Check sheet for the drawn part. Datum: minimum x, y, z corner. Units: mm. A direction names the side the tool comes from. Coordinates: 2 decimals unless noted, no trailing zeros. Write each loop counter-clockwise with the first axis right and the second up, starting at its lowest first coordinate (ties: lowest second). Pieces come first, ordered by that corner, then holes. Notation, with made-up numbers: (47.5, -24.5) -> (77.5, -24.5) arc R18 ccw to (77.5, -10.5) -> close; hole circle Ø4 at (21.5, 80.5). An arc over 180 degrees is marked (long way). Write item = value, one per line. Start each with the question number.
(1) Set-up check for the marked faces 5, 6 and 7: record each of +Z, -Z, +X, -X, +Y, -Y from which the full face is reachable in a straight line by a thin tool's end or side.
(2) Section check A-A (y = 0.75). Record the cut outline in (x, z), plus the area to 3 significant figures.
(3) Mould release check, pull along X, two halves, no side actions. Record for the marked faces 1, 2, 3 and 4: released by +X, released by -X, zero draft, split by the parting line, or undercut.
(4) Gauge pin test, flat ends, axial feed: pin 1 Ø1.5 at (x, z) = (12, 3) entering from -Y; pin 2 Ø0.9 at (y, z) = (1, 4.5) entering from +X; pin 3 Ø1.5 at (y, z) = (1.5, 3) entering from -X. Record the tip position at first contact, or that the pin passes through.
(5) Section check B-B (z = 4.5). Record the cut outline in (x, y), plus the area to 3 significant figures.
(6) Material ranges on probe 1 along X at (y, z) = (1.05, 7.25); probe 2 along Y at (x, z) = (11.5, 1), recorded low to high. Write a range as [from, to].
(7) Section check C-C (x = 13.5). Record the cut outline in (y, z).
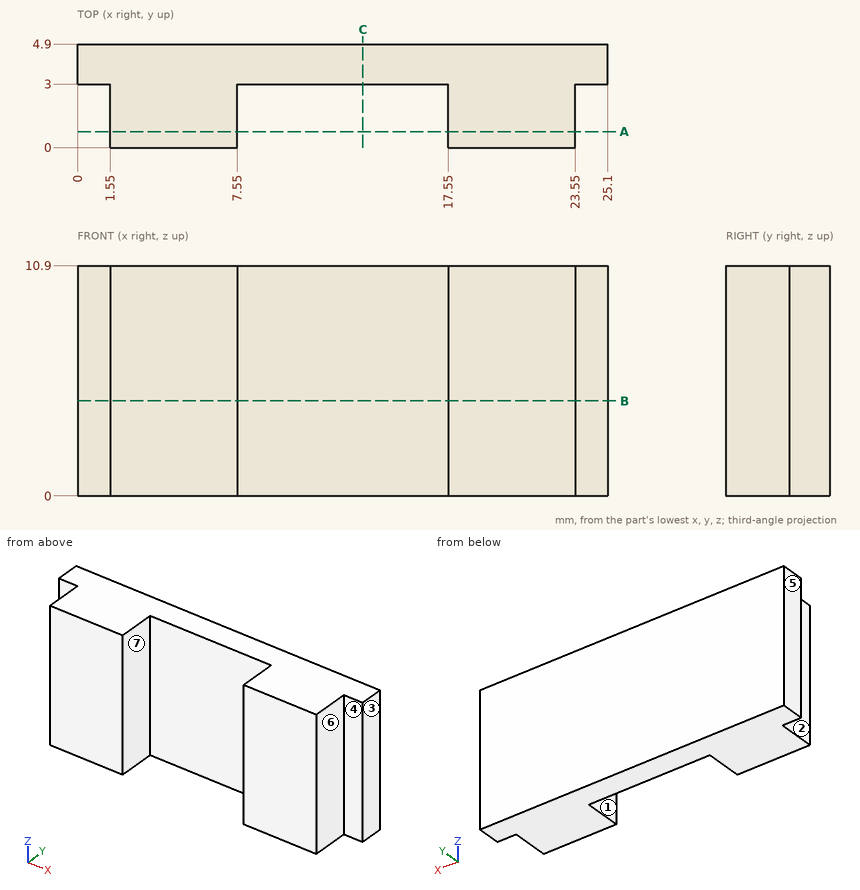
Response:
q1.face_5 = +Z, -Z, -X, +Y, -Y
q1.face_6 = +Z, -Z, +X, -Y
q1.face_7 = +Z, -Z, -Y
q2.outline = (1.55, 0) -> (7.55, 0) -> (7.55, 10.9) -> (1.55, 10.9) -> close; (17.55, 0) -> (23.55, 0) -> (23.55, 10.9) -> (17.55, 10.9) -> close
q2.area = 131 mm2
q3.face_1 = undercut
q3.face_2 = released by -X
q3.face_3 = released by +X
q3.face_4 = zero draft
q4.pin_1 = 3
q4.pin_2 = 23.55
q4.pin_3 = 1.55
q5.outline = (0, 3) -> (1.55, 3) -> (1.55, 0) -> (7.55, 0) -> (7.55, 3) -> (17.55, 3) -> (17.55, 0) -> (23.55, 0) -> (23.55, 3) -> (25.1, 3) -> (25.1, 4.9) -> (0, 4.9) -> close
q5.area = 83.7 mm2
q6.probe_1 = [1.55, 7.55], [17.55, 23.55]
q6.probe_2 = [3, 4.9]
q7.outline = (3, 0) -> (4.9, 0) -> (4.9, 10.9) -> (3, 10.9) -> close
